```python
from build123d import *

# Parameters (mm, degrees)
SKETCH1_W                      = 15.875
SKETCH1_H                      = 22.225
SKETCH1_H_2                    = 50.8
BOSS_EXTRUDE1_DEPTH            = 4.7625
F_3_16_0_1875_DIAMETER_HOLE1_D = 4.7625
SKETCH5_W                      = 4.7625
SKETCH5_H                      = 15.875
BOSS_EXTRUDE2_DEPTH            = 4.7625
FILLET1_R                      = 6.35
SKETCH7_W                      = 19.05
SKETCH7_H                      = 10.16
CUT_EXTRUDE1_DEPTH             = 78.7875


with BuildPart() as part:
    # Sketch1 → Boss-Extrude1 (new body)
    with BuildSketch(Plane(origin=(0, 0, 0), x_dir=(0, 0, -1), z_dir=(1, 0, 0))):
        with Locations((0, 36.5125)):
            Rectangle(SKETCH1_W, SKETCH1_H)
        Rectangle(SKETCH1_W, SKETCH1_H_2)
    extrude(amount=BOSS_EXTRUDE1_DEPTH)

    # 3/16 (0.1875) Diameter Hole1 (through all)
    with Locations(Plane(origin=(4.7625, 0, 0), x_dir=(0, 0, -1), z_dir=(1, 0, 0))):
        with Locations((0, -15.875), (0, 15.875)):
            Hole(F_3_16_0_1875_DIAMETER_HOLE1_D / 2)

    # Sketch5 → Boss-Extrude2 (add)
    with BuildSketch(Plane(origin=(0, 47.625, 0), x_dir=(1, 0, 0), z_dir=(0, 1, 0))):
        Polygon((-20.6375, -7.9375), (0, -7.9375), (0, 7.9375), (4.7625, 7.9375), (4.7625, 28.575), (-20.6375, 28.575), align=None)
        with Locations((2.38125, 0)):
            Rectangle(SKETCH5_W, SKETCH5_H)
    extrude(amount=BOSS_EXTRUDE2_DEPTH)

    # Fillet1
    fillet1_edges = [part.edges().sort_by_distance(p)[0] for p in [
        (2.38125, -25.4, 7.9375),
        (2.38125, -25.4, -7.9375),
    ]]
    fillet(fillet1_edges, radius=FILLET1_R)

    # Sketch7 → Cut-Extrude1 (cut, through all)
    with BuildSketch(Plane(origin=(0, 52.3875, 0), x_dir=(1, 0, 0), z_dir=(0, 1, 0))):
        with Locations((-7.9375, 19.685)):
            Rectangle(SKETCH7_W, SKETCH7_H)
    extrude(amount=-CUT_EXTRUDE1_DEPTH, mode=Mode.SUBTRACT)


solid = part.part
```
Build history of the part. All positions in model axes, mm. A direction names the side the tool comes from. Round coordinates to 2 decimals unless told otherwise and drop trailing zeros. Order: outer loops, then holes, each group sorted by start corner. A loop starts at its lowest first (then second) coordinate and runs counter-clockwise, first axis right, second up. Notation, with made-up numbers: (-3, 20.25) - (15, 20.25) arc R29 ccw to (15, 58.25) - close; hole circle Ø2 at (77.25, -38.75). An arc over 180 degrees is marked (long way). Use a Markdown table: item, result.
1) Saw through at B-B on z = 0. Write the cut outline in (x, y) (1 decimal), and give its area (3 significant figures).
Recorded:
| item | result |
|---|---|
| outline | (-20.6, 47.6) - (0, 47.6) - (0, 18.3) - (4.8, 18.3) - (4.8, 52.4) - (-20.6, 52.4) - close; (0, -25.4) - (4.8, -25.4) - (4.8, -18.3) - (0, -18.3) - close; (0, -13.5) - (4.8, -13.5) - (4.8, 13.5) - (0, 13.5) - close |
| area | 423 mm² |
2) Saw through at A-A on x = -9.5. Write the cut outline in (y, z) (1 decimal).
Recorded:
| item | result |
|---|---|
| outline | (47.6, -28.6) - (52.4, -28.6) - (52.4, -24.8) - (47.6, -24.8) - close; (47.6, -14.6) - (52.4, -14.6) - (52.4, 7.9) - (47.6, 7.9) - close |
3) Saw through at D-D on y = -6. Write the cut outline in (x, z).
Recorded:
| item | result |
|---|---|
| outline | (0, -7.94) - (4.76, -7.94) - (4.76, 7.94) - (0, 7.94) - close |
4) Tool access for faces 4 (the face through (0, 12, 0)), 5 (the face through (1.588, 50, -20)), 6 (the face through (2, 14, -7.938)): list every direction of +Z, -Z, +X, -X, +Y, -Y with a clear straight run to the whole face (end or side of a thin tool).
Recorded:
| item | result |
|---|---|
| face 4 | +Z, -Z, -X, -Y |
| face 5 | +Y, -Y |
| face 6 | -Z, +X, -X, -Y |
5) Flat gauge pins, fed straight in: pin 1 Ø12.5 at (y, z) = (5.5, -0.5) entering from -X; pin 2 Ø2.5 at (x, y) = (2, 5.5) entering from -Z. Where does each tip first touch, or does it go through?
Recorded:
| item | result |
|---|---|
| pin 1 | stops at x = 0 |
| pin 2 | stops at z = -7.94 |
6) Saw through at C-C on y = 17. Write the cut outline in (x, z).
Recorded:
| item | result |
|---|---|
| outline | (0, -7.94) - (4.76, -7.94) - (4.76, -2.1) - (0, -2.1) - close; (0, 2.1) - (4.76, 2.1) - (4.76, 7.94) - (0, 7.94) - close |
7) Pull direction X, two halves, no side cores. Call faces 1 (the face through (-11, 47.625, -11)), 2 (the face through (-17.462, 50, -20)), 3 (the face through (4.762, 13, -2)): pulls with the +X half, pulls with the -X half, needs draft (parallel to the pull), parting line crosses it, or undercut.
Recorded:
| item | result |
|---|---|
| face 1 | needs draft |
| face 2 | undercut |
| face 3 | pulls with the +X half |
8) Wall check: L1, parallel to Y at x = 3.8, z = 0; L2, parallel to Y at x = -7.25, z = -9 (1 decimal); L3, parallel to X at y = -11, z = -6. Give the ranges that are in metal, low to high.
Recorded:
| item | result |
|---|---|
| L1 | y = -25.4 to -18.26, -13.49 to 13.49, 18.26 to 52.39 |
| L2 | y = 47.6 to 52.4 |
| L3 | x = 0 to 4.76 |
